Part model, mm, in its own coordinate system. Face numbers are marked on the shaded views. A direction names the side the tool comes from. Coordinates: 2 decimals unless noted, no trailing zeros. Order: outer loops, then holes, each group sorted by start corner. A loop starts at its lowest first (then second) coordinate and runs counter-clockwise, first axis right, second up.
from build123d import *

# Parameters (mm, degrees)
BOX008_W                  = 200
BOX008_H                  = 200
BOX008_DEPTH              = 10
CYLINDER014_R             = 4
CYLINDER014_DEPTH         = 4
CYLINDER015_R             = 2.4
CYLINDER015_DEPTH         = 10
FUSION014_PLACEMENT_ANGLE = 90
CYLINDER016_R             = 4
CYLINDER016_DEPTH         = 4
CYLINDER017_R             = 2.4
CYLINDER017_DEPTH         = 10
FUSION015_PLACEMENT_ANGLE = 90
BOX007_W                  = 120
BOX007_H                  = 8
BOX007_DEPTH              = 10
CYLINDER012_R             = 4
CYLINDER012_DEPTH         = 10
CYLINDER013_R             = 4
CYLINDER013_DEPTH         = 10
CYLINDER010_R             = 2.4
CYLINDER010_DEPTH         = 100
CYLINDER011_R             = 2.4
CYLINDER011_DEPTH         = 100
EXTRUDE_DEPTH             = 2.4
LINK003_PLACEMENT_ANGLE   = 90
BOX006_W                  = 11
BOX006_H                  = 10
BOX006_DEPTH              = 8
FUSION010_PLACEMENT_ANGLE = 180
BOX005_W                  = 10
BOX005_H                  = 10
BOX005_DEPTH              = 8
LINK002_SCALE_SCALE       = 1.1
LINK002_PLACEMENT_ANGLE   = 90
CYLINDER009_R             = 25.5
CYLINDER009_DEPTH         = 10
BOX004_W                  = 74
BOX004_H                  = 70
BOX004_DEPTH              = 10
BOX010_W                  = 10
BOX010_H                  = 0.2
BOX010_DEPTH              = 10
BOX011_W                  = 10
BOX011_H                  = 0.2
BOX011_DEPTH              = 10
BOX012_W                  = 10
BOX012_H                  = 0.2
BOX012_DEPTH              = 10
BOX013_W                  = 10
BOX013_H                  = 0.2
BOX013_DEPTH              = 10


with BuildPart() as cube008:
    # Box008 → Box008 (new body)
    with BuildSketch(Plane(origin=(-100, 0, 0), x_dir=(1, 0, 0), z_dir=(0, 0, 1))):
        with Locations((100, 100)):
            Rectangle(BOX008_W, BOX008_H)
    extrude(amount=BOX008_DEPTH)


with BuildPart() as cylinder014:
    # Cylinder014 → Cylinder014 (new body)
    with BuildSketch(Plane.XY):
        Circle(CYLINDER014_R)
    extrude(amount=CYLINDER014_DEPTH)


with BuildPart() as fusion014:
    # Cylinder015 → Cylinder015 (new body)
    with BuildSketch(Plane.XY):
        Circle(CYLINDER015_R)
    extrude(amount=CYLINDER015_DEPTH)

    # Fusion014: union Cylinder014
    add(cylinder014.part)


with BuildPart() as fusion014_1:
    # Fusion014 placement: moved
    add(fusion014.part.moved(Location((-50, -27, 5))).rotate(Axis((-50, -27, 5), (1, 0, 0)), FUSION014_PLACEMENT_ANGLE))


with BuildPart() as cylinder016:
    # Cylinder016 → Cylinder016 (new body)
    with BuildSketch(Plane.XY):
        Circle(CYLINDER016_R)
    extrude(amount=CYLINDER016_DEPTH)


with BuildPart() as fusion016:
    # Cylinder017 → Cylinder017 (new body)
    with BuildSketch(Plane.XY):
        Circle(CYLINDER017_R)
    extrude(amount=CYLINDER017_DEPTH)

    # Fusion015: union Cylinder016
    add(cylinder016.part)


with BuildPart() as fusion016_1:
    # Fusion015 placement: moved
    add(fusion016.part.moved(Location((50, -27, 5))).rotate(Axis((50, -27, 5), (1, 0, 0)), FUSION015_PLACEMENT_ANGLE))

    # Fusion016: union Fusion014
    add(fusion014_1.part)


with BuildPart() as cut009:
    # Box007 → Box007 (new body)
    with BuildSketch(Plane(origin=(-60, -35, 0), x_dir=(1, 0, 0), z_dir=(0, 0, 1))):
        with Locations((60, 4)):
            Rectangle(BOX007_W, BOX007_H)
    extrude(amount=BOX007_DEPTH)

    # Cut009: cut Fusion016
    add(fusion016_1.part, mode=Mode.SUBTRACT)


with BuildPart() as cylinder012:
    # Cylinder012 → Cylinder012 (new body)
    with BuildSketch(Plane(origin=(31, 35, 5), x_dir=(1, 0, 0), z_dir=(0, -1, 0))):
        Circle(CYLINDER012_R)
    extrude(amount=CYLINDER012_DEPTH)


with BuildPart() as fusion013:
    # Cylinder013 → Cylinder013 (new body)
    with BuildSketch(Plane(origin=(-31, 35, 5), x_dir=(1, 0, 0), z_dir=(0, -1, 0))):
        Circle(CYLINDER013_R)
    extrude(amount=CYLINDER013_DEPTH)

    # Fusion013: union Cylinder012
    add(cylinder012.part)


with BuildPart() as cylinder010:
    # Cylinder010 → Cylinder010 (new body)
    with BuildSketch(Plane(origin=(-31, 94, 5), x_dir=(1, 0, 0), z_dir=(0, -1, 0))):
        Circle(CYLINDER010_R)
    extrude(amount=CYLINDER010_DEPTH)


with BuildPart() as fusion012:
    # Cylinder011 → Cylinder011 (new body)
    with BuildSketch(Plane(origin=(31, 94, 5), x_dir=(1, 0, 0), z_dir=(0, -1, 0))):
        Circle(CYLINDER011_R)
    extrude(amount=CYLINDER011_DEPTH)

    # Fusion012: union Cylinder010
    add(cylinder010.part)


with BuildPart() as din934_m006:
    # Sketch → Extrude (new body)
    with BuildSketch(Plane.XY):
        Polygon((-3.005, 0), (-1.5025, -2.602406), (1.5025, -2.602406), (3.005, 0), (1.5025, 2.602406), (-1.5025, 2.602406), align=None)
    extrude(amount=EXTRUDE_DEPTH)


with BuildPart() as din934_m008:
    # Link003 base: copy of DIN934_M006
    add(din934_m006.part)


with BuildPart() as din934_m008_1:
    # Link003 placement: moved
    add(din934_m008.part.moved(Location((-31, -3, 5))).rotate(Axis((-31, -3, 5), (1, 0, 0)), LINK003_PLACEMENT_ANGLE))


with BuildPart() as fusion010:
    # Box006 → Box006 (new body)
    with BuildSketch(Plane(origin=(-39, -15, 1), x_dir=(1, 0, 0), z_dir=(0, 0, 1))):
        with Locations((5.5, 5)):
            Rectangle(BOX006_W, BOX006_H)
    extrude(amount=BOX006_DEPTH)

    # Fusion010: union DIN934_M008
    add(din934_m008_1.part)


with BuildPart() as fusion010_1:
    # Fusion010 placement: moved
    add(fusion010.part.moved(Location((0, 0, 10))).rotate(Axis((0, 0, 10), (0, 1, 0)), FUSION010_PLACEMENT_ANGLE))


with BuildPart() as cube005:
    # Box005 → Box005 (new body)
    with BuildSketch(Plane(origin=(-37, -15, 1), x_dir=(1, 0, 0), z_dir=(0, 0, 1))):
        with Locations((5, 5)):
            Rectangle(BOX005_W, BOX005_H)
    extrude(amount=BOX005_DEPTH)


with BuildPart() as fusion011:
    # Link002 base: copy of DIN934_M006
    add(din934_m006.part)


with BuildPart() as fusion011_1:
    # Link002 scale: moved
    add(fusion011.part.scale(LINK002_SCALE_SCALE))


with BuildPart() as fusion011_2:
    # Link002 placement: moved
    add(fusion011_1.part.moved(Location((-31, -3, 5))).rotate(Axis((-31, -3, 5), (1, 0, 0)), LINK002_PLACEMENT_ANGLE))

    # Fusion009: union Cube005
    add(cube005.part)

    # Fusion011: union Fusion010
    add(fusion010_1.part)


with BuildPart() as cylinder009:
    # Cylinder009 → Cylinder009 (new body)
    with BuildSketch(Plane.XY):
        Circle(CYLINDER009_R)
    extrude(amount=CYLINDER009_DEPTH)


with BuildPart() as lowerpart:
    # Box004 → Box004 (new body)
    with BuildSketch(Plane(origin=(-37, -35, 0), x_dir=(1, 0, 0), z_dir=(0, 0, 1))):
        with Locations((37, 35)):
            Rectangle(BOX004_W, BOX004_H)
    extrude(amount=BOX004_DEPTH)

    # Cut005: cut Cylinder009
    add(cylinder009.part, mode=Mode.SUBTRACT)

    # Cut006: cut Fusion011
    add(fusion011_2.part, mode=Mode.SUBTRACT)

    # Cut007: cut Fusion012
    add(fusion012.part, mode=Mode.SUBTRACT)

    # Cut008: cut Fusion013
    add(fusion013.part, mode=Mode.SUBTRACT)

    # Fusion017: union Cut009
    add(cut009.part)

    # Cut011: cut Cube008
    add(cube008.part, mode=Mode.SUBTRACT)


with BuildPart() as cube010:
    # Box010 → Box010 (new body)
    with BuildSketch(Plane(origin=(-37, -5, 0), x_dir=(1, 0, 0), z_dir=(0, 0, 1))):
        with Locations((5, 0.1)):
            Rectangle(BOX010_W, BOX010_H)
    extrude(amount=BOX010_DEPTH)


with BuildPart() as cube011:
    # Box011 → Box011 (new body)
    with BuildSketch(Plane(origin=(-37, -3, 0), x_dir=(1, 0, 0), z_dir=(0, 0, 1))):
        with Locations((5, 0.1)):
            Rectangle(BOX011_W, BOX011_H)
    extrude(amount=BOX011_DEPTH)


with BuildPart() as cube012:
    # Box012 → Box012 (new body)
    with BuildSketch(Plane(origin=(27, -3, 0), x_dir=(1, 0, 0), z_dir=(0, 0, 1))):
        with Locations((5, 0.1)):
            Rectangle(BOX012_W, BOX012_H)
    extrude(amount=BOX012_DEPTH)


with BuildPart() as lowerpart_print:
    # Box013 → Box013 (new body)
    with BuildSketch(Plane(origin=(27, -5, 0), x_dir=(1, 0, 0), z_dir=(0, 0, 1))):
        with Locations((5, 0.1)):
            Rectangle(BOX013_W, BOX013_H)
    extrude(amount=BOX013_DEPTH)

    # Fusion018: union Cube010, Cube011, Cube012
    add(cube010.part)
    add(cube011.part)
    add(cube012.part)

    # Fusion019: union LowerPart
    add(lowerpart.part)


solid = lowerpart_print.part
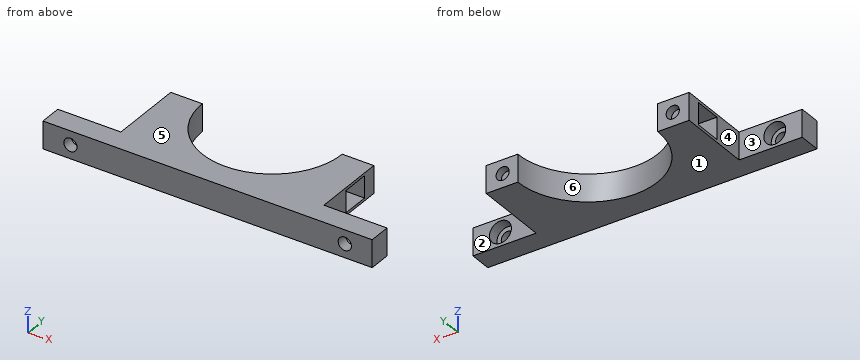
Q1. Cut at B-B on x = 50. Write the cut outline in (y, z), and give its area (3 significant figures).
Results list:
outline: (-35, 0) - (-27, 0) - (-27, 1) - (-31, 1) - (-31, 2.6) - (-35, 2.6) - close; (-35, 7.4) - (-31, 7.4) - (-31, 9) - (-27, 9) - (-27, 10) - (-35, 10) - close
area: 28.8 mm2
Q2. Pin check, flat tips, straight feed: pin 1 Ø8 at (x, y) = (0, -20) entering from -Z; pin 2 Ø3 at (y, z) = (-16, 6) entering from -X; pin 3 Ø4 at (x, z) = (48.5, 6.5) entering from +Y. Stop position of each tip, or through.
Results list:
pin 1: passes through
pin 2: stops at x = -37
pin 3: stops at y = -27
Q3. Cut at A-A on x = 31. Write the cut outline in (y, z).
Results list:
outline: (-35, 0) - (0, 0) - (0, 2.6) - (-2.8, 2.6) - (-2.8, 7.4) - (0, 7.4) - (0, 10) - (-35, 10) - close; hole (-15, 1) - (-5, 1) - (-5, 9) - (-15, 9) - close; hole (-4.8, 2.4) - (-3, 2.4) - (-3, 7.6) - (-4.8, 7.6) - close
Q4. Mould opens along X. For the marked faces 4, 5 and 6 say: pulls with the +X half, pulls with the -X half, needs draft (parallel to the pull), parting line crosses it, or undercut.
Results list:
face 4: pulls with the -X half
face 5: needs draft
face 6: undercut
Q5. Which spindle directions (+Z, -Z, +X, -X, +Y, -Y) get a long thin tool onto all of the face, cutting with end or side? Do the marked faces 1, 2 and 3. Say none if no direction does.
Results list:
face 1: -Z, +X, -X, +Y, -Y
face 2: +Z, -Z, +X, +Y
face 3: +Z, -Z, -X, +Y
Q6. Cut at D-D on x = -2. Write the cut outline in (y, z), and give its area (3 significant figures).
Results list:
outline: (-35, 0) - (-25.42, 0) - (-25.42, 10) - (-35, 10) - close
area: 95.8 mm2
Q7. Wall check: line 1 along Z through (x, y) = (-50, -34.05); line 2 along X through (y, z) = (-2.1, 5); line 3 along Z through (x, y) = (50, -28). Give the ranges that are in metal, low to high.
Results list:
line 1: z = 0 to 2.6, 7.4 to 10
line 2: x = -37 to -33.4, -28.6 to -25.41, 25.41 to 28.6, 33.4 to 37
line 3: z = 0 to 1, 9 to 10
Q8. Cut at C-C on y = -29. Write the cut outline in (x, z), and give its area (3 significant figures).
Results list:
outline: (-60, 0) - (60, 0) - (60, 10) - (-60, 10) - close; hole circle Ø8 at (-50, 5); hole circle Ø8 at (50, 5)
area: 1,100 mm2
